Part model, mm, in its own coordinate system. A direction names the side the tool comes from. Coordinates: 2 decimals unless noted, no trailing zeros. Order: outer loops, then holes, each group sorted by start corner. A loop starts at its lowest first (then second) coordinate and runs counter-clockwise, first axis right, second up. Notation, with made-up numbers: (33, -33) - (67, -33) arc R21 ccw to (67, -10) - close; hole circle Ø1 at (55.5, 56.5). An arc over 180 degrees is marked (long way). Use a Markdown table: item, result. Add a question column.
1) Tool access for faces 1 (the face through (-2, 0, 1.5)), 2 (the face through (9.2, 0, 0)), 3 (the face through (4.26, 0.54, 2.44)): list every direction of +Z, -Z, +X, -X, +Y, -Y with a clear straight run to the whole face (end or side of a thin tool).
2) Drop flat-ended pins along their axis: P1, Ø1, axis at x = 8, z = 1, coming from the -Y side; P2, Ø1.4, axis at x = -2, y = 0, coming from the +Z side; P3, Ø4, axis at x = 3.5, y = 3.5, coming from the +Z side; P4, Ø0.9, axis at x = -2, y = 0, coming from the -Z side. Give the stop position or say it passes through.
3) Saw through at A-A on y = 0. List the corners of the cut face in (x, z), then the cut area to 3 significant figures.
4) Saw through at B-B on x = 1.5. List the corners of the cut face in (y, z), then the cut area to 3 significant figures.
5) Two-plate mould, pull along Z, no slides. Class faces 4 (the face through (-1.863, 1.293, 0.76)), 5 (the face through (-2.8, 0, 2)), 6 (the face through (-2.65, -4.77, -1.5)): +Z half, -Z half, draft (parallel to the pull), parting line (faces both ways), or undercut.
6) Wall check: L1, parallel to Z at x = 3, y = 0; L2, parallel to X at y = 1, z = -0.5; L3, parallel to Z at x = -1.75, y = -0.5. Give the ranges that are in metal, low to high. Write a range as [from, to].
```python
from build123d import *

# Parameters (mm, degrees)
CUT_EXTRUDE1_DEPTH = 1.9


with BuildPart() as part:
    # Sketch1 → Revolve1 (revolve)
    with BuildSketch(Plane.XY):
        Polygon((0, -2.5), (8.4, -2.5), (9.2, -1.7), (9.2, 0), (-2.8, 0), (-2.8, -5), (-2.5, -5), align=None)
    revolve(axis=Axis((-2.8, 0, 0), (1, 0, 0)))

    # Sketch2 → Cut-Extrude1 (cut)
    with BuildSketch(Plane.ZY.offset(2.8)):
        Polygon((0, 1.732050808), (-1.5, 0.866025404), (-1.5, -0.866025404), (0, -1.732050808), (1.5, -0.866025404), (1.5, 0.866025404), align=None)
    extrude(amount=-CUT_EXTRUDE1_DEPTH, mode=Mode.SUBTRACT)


solid = part.part
```
Results are:
| question | item | result |
|---|---|---|
| 1 | face 1 | -X |
| 1 | face 2 | +Z, -Z, +X, +Y, -Y |
| 1 | face 3 | +X |
| 2 | P1 | y = -2.45 |
| 2 | P2 | z = 5 |
| 2 | P3 | z = 2 |
| 2 | P4 | z = -4.95 |
| 3 | outline | (-2.8, -5) - (-2.5, -5) - (0, -2.5) - (8.4, -2.5) - (9.2, -1.7) - (9.2, 1.7) - (8.4, 2.5) - (0, 2.5) - (-2.5, 5) - (-2.8, 5) - (-2.8, 1.5) - (-0.9, 1.5) - (-0.9, -1.5) - (-2.8, -1.5) - close |
| 3 | area | 61.4 mm2 |
| 4 | outline | circle Ø5 at (0, 0) |
| 4 | area | 19.6 mm2 |
| 5 | face 4 | undercut |
| 5 | face 5 | draft |
| 5 | face 6 | parting line |
| 6 | L1 | [-2.5, 2.5] |
| 6 | L2 | [-0.9, 9.2] |
| 6 | L3 | [-4.22, -1.5], [1.5, 4.22] |
